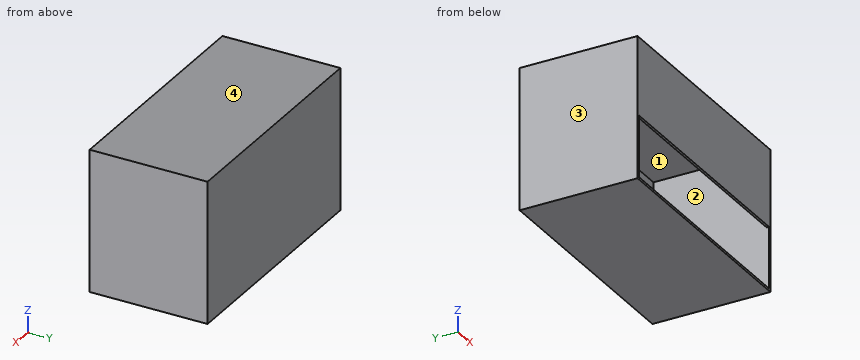
Autodesk Fusion 360 part; units mm, degrees
sketch "Sketch1" plane through (0, 0, 0) normal (0, 0, 1) x (1, 0, 0)
  line L0 (-50, -25) -> (50, -25)
  line L1 (50, -25) -> (50, 25)
  line L2 (50, 25) -> (-50, 25)
  line L3 (-50, 25) -> (-50, -25)
extrude "Extrude1" add sketch "Sketch1" along normal blind 1
sketch "Sketch2" plane through (0, 0, 1) normal (0, 0, 1) x (-1, 0, 0)
  line L0 (50, -25) -> (50, 25)
  line L1 (50, 25) -> (-50, 25)
  line L2 (-50, 25) -> (-50, -25)
  line L3 (-50, -25) -> (50, -25)
  line L4 (49, 24) -> (-49, 24)
  line L5 (-49, 24) -> (-49, -24)
  line L6 (-49, -24) -> (49, -24)
  line L7 (49, -24) -> (49, 24)
  line L8 (49, 24) -> (49, 25)
  line L9 (-49, 24) -> (-49, 25)
  dimension "d3" = -1
extrude "Extrude2" add sketch "Sketch2" along normal blind 59 contours L0 L1 L2 L3 L5 L6 L7 L8 L9
sketch "Sketch3" plane through (0, 0, 60) normal (0, 0, 1) x (-1, 0, 0)
  line L0 (-49, -24) -> (-49, 25)
  line L1 (-49, 25) -> (-50, 25)
  line L2 (-50, 25) -> (-50, -25)
  line L3 (-50, -25) -> (50, -25)
  line L4 (50, -25) -> (50, 25)
  line L5 (50, 25) -> (49, 25)
  line L6 (49, 25) -> (49, -24)
  line L7 (49, -24) -> (-49, -24)
  line L8 (50, -25) -> (-50, -25)
  line L9 (-50, -25) -> (-50, 25)
  line L10 (-50, 25) -> (50, 25)
  line L11 (50, 25) -> (50, -25)
extrude "Extrude3" add sketch "Sketch3" against normal blind 1 contours L0 L6 L7 L10
sketch "Sketch4" plane through (0, 0, 59) normal (0, 0, -1) x (1, 0, 0)
  line L0 (-49, -24) -> (49, -24)
  line L1 (49, -24) -> (49, 25)
  line L2 (49, 25) -> (-49, 25)
  line L3 (-49, 25) -> (-49, -24)
  line L4 (-49, 25) -> (-49, 24)
  line L5 (-49, 24) -> (49, 24)
  dimension "d8" = 1
extrude "Extrude4" add sketch "Sketch4" along normal blind 32 contours L1 L2 L3 L4 L5
For this review, take the finished solid that the model builds, in its own axes (mm). Face numbers are marked on the shaded views. Round coordinates to 2 decimals unless told otherwise and drop trailing zeros. Write each loop counter-clockwise with the first axis right and the second up, starting at its lowest first coordinate (ties: lowest second). Pieces come first, ordered by that corner, then holes. Notation, with made-up numbers: (40.5, 44.25) -> (82.5, 44.25) arc R30 cw to (82.5, 69.25) -> close; hole circle Ø6 at (39, 12). An arc over 180 degrees is marked (long way). Use one line per item in the form item = value.
Q1. To check wall thickness, follow probe 1 along Z at (x, y) = (1.5, 7); probe 2 along Y at (x, z) = (43.5, 48); probe 3 along X at (y, z) = (19.5, 48.5). State the ranges of each line that lie inside material, in increasing order. Write a range as from..to.
Resolved:
probe_1 = 0..1, 59..60
probe_2 = -25..-24, 24..25
probe_3 = -50..-49, 49..50
Q2. Consider section C-C (x = -23). State the section outline as (y, z) points.
Resolved:
outline = (-25, 0) -> (25, 0) -> (25, 60) -> (-25, 60) -> (-25, 27) -> (-24, 27) -> (-24, 59) -> (24, 59) -> (24, 1) -> (-25, 1) -> close
Q3. Consider section B-B (z = 44.5). State the section outline as (x, y) points.
Resolved:
outline = (-50, -25) -> (50, -25) -> (50, 25) -> (-50, 25) -> close; hole (-49, -24) -> (49, -24) -> (49, 24) -> (-49, 24) -> close
Q4. Consider section D-D (z = 21). State the section outline as (x, y) points, then the cut area to 3 significant figures.
Resolved:
outline = (-50, -25) -> (-49, -25) -> (-49, 24) -> (49, 24) -> (49, -25) -> (50, -25) -> (50, 25) -> (-50, 25) -> close
area = 198 mm²
Q5. The part is to be moulded in two halves that separate along X. For the marked faces 1, 2, 3 and 4, say which applies: released by +X, released by -X, zero draft, split by the parting line, or undercut.
Resolved:
face_1 = undercut
face_2 = undercut
face_3 = released by -X
face_4 = zero draft
Q6. Consider section A-A (y = 15.5). State the section outline as (x, z) points, then the cut area to 3 significant figures.
Resolved:
outline = (-50, 0) -> (50, 0) -> (50, 60) -> (-50, 60) -> close; hole (-49, 1) -> (49, 1) -> (49, 59) -> (-49, 59) -> close
area = 316 mm²
Q7. Clearance check with a flat-ended pin moving along its axis: pin 1 Ø24 at (x, y) = (2.5, 3) entering from -Z. State where the tip first meets the part, or that it passes through.
Resolved:
pin_1 = 0
